Model file for the job. Use its own axes, mm. Give positions to 0.01 mm unless a question says otherwise; leave off trailing zeros. Write each loop counter-clockwise with the first axis right and the second up, starting at its lowest first coordinate (ties: lowest second). Pieces come first, ordered by that corner, then holes. Notation, with made-up numbers: (61, 62.5) - (119, 62.5) arc R28 cw to (119, 81.5) - close; hole circle Ø10 at (49.5, 23). An arc over 180 degrees is marked (long way). Use CSV: the item, a comma, the result in double quotes.
Autodesk Inventor part; units mm, degrees
ref_plane "Arbeitsebene7" through (120, 40, 0) normal (0, 1, 0) x (-1, 0, 0)
ref_plane "Arbeitsebene8" through (120, -40, 0) normal (0, 1, 0) x (-1, 0, 0)
ref_plane "Arbeitsebene10" through (20, -140, 0) normal (0, -1, 0) x (1, 0, 0)
sketch "Basis" plane through (0, 0, 0) normal (0, 0, 1) x (1, 0, 0)
  line L0 (0, 150) -> (0, -150)
  line L1 (-79.5351, 0) -> (153.2558, 0)
  line L2 (0, -282) -> (0, 222)
  line L3 (30, -50) -> (30, -210)
  line L4 (0, -200) -> (20, -200)
  line L5 (0, -40) -> (120, -40)
  line L6 (0, 40) -> (120, 40)
  line L7 (110, -30) -> (110, 30)
  point P0 (0, 0)
  point P1 (110, 0)
  dimension "d32" = 300
  dimension "d38" = 80
  dimension "d39" = 10
  dimension "d40" = 10
  dimension "d41" = 10
  dimension "d43" = 240
  dimension "d44" = 240
  dimension "d45" = 60
  dimension "d46" = 10
  dimension "d47" = 10
  dimension "d48" = 160
  dimension "d49" = 10
ref_plane "Arbeitsebene7" through (120, 40, 0) normal (0, 1, 0) x (-1, 0, 0)
sketch "Skizze12" plane through (120, 40, 0) normal (0, 1, 0) x (-1, 0, 0)
  line L0 (10, -10) -> (10, -80)
  line L1 (20, -70) -> (120, -70)
  line L2 (120, -100.8) -> (120, 16.8)
  point P0 (120, 0)
  point P1 (10, 0)
  point P2 (10, 0)
  point P3 (10, 0)
  dimension "d50" = 70
  dimension "d51" = 10
  dimension "d80" = 10
  dimension "d81" = 10
ref_plane "Arbeitsebene8" through (120, -40, 0) normal (0, 1, 0) x (-1, 0, 0)
sketch "Skizze13" plane through (120, -40, 0) normal (0, 1, 0) x (-1, 0, 0)
  line L0 (10, -10) -> (10, -80)
  line L1 (10, -10) -> (10, -80)
  line L2 (20, -70) -> (120, -70)
  line L3 (120, -100.8) -> (120, 16.8)
  point P0 (120, 0)
  dimension "d82" = 10
  dimension "d83" = 10
ref_plane "Arbeitsebene9" through (20, -200, 0) normal (0, -1, 0) x (1, 0, 0)
sketch "Skizze14" plane through (20, -200, 0) normal (0, -1, 0) x (1, 0, 0)
  line L0 (10, -10) -> (10, -50)
  point P0 (-20, 0)
  point P1 (10, 0)
  point P2 (10, 0)
  point P3 (10, 0)
  dimension "d52" = 40
  dimension "d53" = 10
ref_plane "Arbeitsebene10" through (20, -140, 0) normal (0, -1, 0) x (1, 0, 0)
sketch "Skizze15" plane through (20, -140, 0) normal (0, -1, 0) x (1, 0, 0)
  line L0 (10, -10) -> (10, -50)
  line L1 (10, -10) -> (10, -50)
  point P0 (-20, 0)
ref_plane "Arbeitsebene12" through (110, 40, -80) normal (1, 0, 0) x (0, 1, 0)
sketch "Skizze16" plane through (110, 40, -80) normal (1, 0, 0) x (0, 1, 0)
  line L0 (-90, 0) -> (10, 0)
  line L1 (10, 0) -> (10, -4)
  line L2 (10, -4) -> (-90, -4)
  line L3 (-90, -4) -> (-90, 0)
  line L4 (-70, 10) -> (-10, 10)
  line L5 (0, 70) -> (0, 0)
  line L6 (-80, 70) -> (-80, 0)
  point P0 (-40, 80)
  dimension "d66" = 4
  dimension "d67" = 10
  dimension "d68" = 10
  dimension "d77" = 10
  dimension "d78" = 10
  dimension "d79" = 10
ref_plane "Arbeitsebene17" through (110, -50, -84) normal (0, 0, 1) x (1, 0, 0)
sketch "Skizze18" plane through (110, -50, -84) normal (0, 0, 1) x (1, 0, 0)
  line L0 (-110, -232) -> (-110, 272)
  line L1 (-189.5351, 50) -> (43.2558, 50)
  line L2 (-19.5, 65.5) -> (-50.5, 65.5) construction
  line L3 (-50.5, 65.5) -> (-50.5, 34.5) construction
  line L4 (-19.5, 65.5) -> (-19.5, 34.5) construction
  line L5 (-19.5, 34.5) -> (-50.5, 34.5) construction
  point P0 (-110, 50)
  point P1 (-35, 50)
  dimension "d69" = 75
  dimension "d70" = 15.5
  dimension "d71" = 15.5
  dimension "d72" = 31
  dimension "d73" = 31
ref_plane "Arbeitsebene18" through (30, -140, -50) normal (1, 0, 0) x (0, 1, 0)
sketch "Skizze19" plane through (30, -140, -50) normal (1, 0, 0) x (0, 1, 0)
  line L0 (10, -4) -> (-70, -4)
  line L1 (-70, -4) -> (-70, 0)
  line L2 (-70, 0) -> (10, 0)
  line L3 (10, 0) -> (10, -4)
  line L4 (-50, 10) -> (-10, 10)
  point P0 (140, 50)
  point P1 (-60, 0)
  point P2 (0, 0)
  dimension "d74" = 4
  dimension "d75" = 10
  dimension "d76" = 10
  dimension "d84" = 10
  dimension "d85" = 10
  dimension "d86" = 10
ref_plane "Arbeitsebene19" through (30, -210, -54) normal (0, 0, 1) x (1, 0, 0)
ref_plane "Arbeitsebene20" through (20, 2.5, 100) normal (0, 0, -1) x (-1, 0, 0)
sketch "Skizze 1" plane through (-280, -73.3, 100) normal (0, 0, 1) x (1, 0, 0)
  line L0 (-20, 13.3) -> (-20, 11.3)
  line L1 (180, 13.3) -> (-20, 13.3)
  line L2 (180, -106.7) -> (-20, -106.7)
  line L3 (-20, -104.7) -> (-20, -106.7)
  line L4 (180, 53.3) -> (180, -146.7)
  line L5 (180, 73.3) -> (180, -166.7)
  line L6 (300, 73.3) -> (300, -166.7)
  line L7 (180, 73.3) -> (182, 73.3)
  line L8 (298, 73.3) -> (300, 73.3)
  line L9 (300, -166.7) -> (298, -166.7)
  line L10 (182, -166.7) -> (180, -166.7)
  line L11 (-20, -106.7) -> (-20, 13.3)
  line L12 (180, 13.3) -> (-20, 13.3)
  line L13 (180, 13.3) -> (180, 73.3)
  line L14 (180, 73.3) -> (300, 73.3)
  line L15 (300, -166.7) -> (300, 73.3)
  line L16 (300, -166.7) -> (180, -166.7)
  line L17 (180, -166.7) -> (180, -106.7)
  line L18 (180, -106.7) -> (-20, -106.7)
extrude "Extrusion3" add sketch "Skizze 1" along normal blind 10
sketch "Skizze23" plane through (20, -242.5, 0) normal (1, 0, 0) x (0, 0, -1)
  line L0 (0, 245) -> (0, 0)
  line L1 (-100, 245) -> (0, 245)
  line L2 (0, 0) -> (-100, 0)
  line L3 (-100, 0) -> (-100, 245)
  line L4 (-100, 245) -> (0, 245)
  line L5 (0, 245) -> (0, 0)
  point P0 (0, 242.5)
extrude "Extrusion4" cut sketch "Skizze23" against normal through all
sketch "Skizze20" plane through (30, -210, 100) normal (0, 0, 1) x (1, 0, 0)
  line L0 (0, 80) -> (0, 0)
  line L1 (-217.5819, 99.185) -> (-324.0785, 99.185) construction
  line L2 (-223.1225, 80.815) -> (-333.4519, 80.815) construction
  line L3 (-289.05, 125.855) -> (-289.05, 54.145) construction
  line L4 (-254.68, 148.5562) -> (-254.68, 51.145) construction
  line L5 (-44.2587, 170.5) -> (-93.3542, 170.5) construction
  line L6 (-85.5, 183.5563) -> (-85.5, 134.1968) construction
  line L7 (-97.1508, 139.5) -> (-51.7506, 139.5) construction
  line L8 (-54.5, 132.7748) -> (-54.5, 177.4853) construction
  line L9 (-327.4713, 90) -> (-3.4708, 90) construction
  line L10 (-70, 254.6178) -> (-70, -44.1957) construction
  line L11 (-130, 210) -> (-10, 210) construction
  line L12 (-330, 30) -> (-330, 150) construction
  circle A0 centre (-289.05, 99.185) radius 1.35
  circle A1 centre (-254.68, 99.185) radius 1.35
  circle A2 centre (-254.68, 80.815) radius 1.35
  circle A3 centre (-289.05, 80.815) radius 1.35
  circle A4 centre (-280, 90) radius 3
  circle A5 centre (-85.5, 170.5) radius 1.5
  circle A6 centre (-85.5, 139.5) radius 1.5
  circle A7 centre (-54.5, 139.5) radius 1.5
  circle A8 centre (-54.5, 170.5) radius 1.5
  circle A9 centre (-70, 155) radius 11
  point P0 (-30, 210)
  point P1 (-70, 210)
  point P2 (-330, 90)
  point P3 (-289.05, 90)
  dimension "d102" = 2.7
  dimension "d103" = 2.7
  dimension "d104" = 2.7
  dimension "d105" = 2.7
  dimension "d106" = 6
  dimension "d107" = 9.05
  dimension "d108" = 9.185
  dimension "d109" = 18.37
  dimension "d111" = 34.37
  dimension "d112" = 50
  dimension "d113" = 31
  dimension "d114" = 31
  dimension "d115" = 15.5
  dimension "d116" = 15.5
  dimension "d117" = 55
  dimension "d118" = 3
  dimension "d119" = 3
  dimension "d120" = 3
  dimension "d121" = 3
  dimension "d122" = 22
extrude "Extrusion5" cut sketch "Skizze20" along normal through all
ref_plane "Arbeitsebene21" through (-297.4713, -120, 100) normal (0, 1, 0) x (1, 0, 0)
mirror "Spiegeln1" about plane through (-297.4713, -120, 100) normal (0, 1, 0) of "Extrusion5"
fillet "Rundung1" radius 2 6 edges at (20, -240, 105) (20, 0, 105) (-100, 0, 105) (-300, -60, 105) (-300, -180, 105) (-100, -240, 105)
equation "\"d38\" = Bas_Haupt_Breite"
equation "\"d39\" = 0.5 * Alu_Prof"
equation "\"d40\" = d39"
equation "\"d41\" = d39"
equation "\"d43\" = Bas_Haupt_Länge + Alu_Prof"
equation "\"d44\" = d43"
equation "\"d45\" = Bas_Ver_Breite"
equation "\"d46\" = d39"
equation "\"d47\" = d39"
equation "\"d48\" = Bas_Ver_Länge"
equation "\"d49\" = d39"
equation "\"d50\" = Bas_Haupt_Höhe - 0.5 * Alu_Prof"
equation "\"d80\" = d51"
equation "\"d81\" = d51"
equation "\"d82\" = d81"
equation "\"d83\" = d81"
equation "\"d52\" = GM_Halt_Höhe - 0.5 * Alu_Prof"
equation "\"d66\" = Bas_Haupt_Plat_Höhe"
equation "\"d67\" = 0.5 * Alu_Prof"
equation "\"d68\" = d67"
equation "\"d77\" = d68"
equation "\"d78\" = d68"
equation "\"d79\" = d68"
equation "\"d70\" = 0.5 * SM_Schrauben_Pos_Abstand"
equation "\"d72\" = SM_Schrauben_Pos_Abstand"
equation "\"d73\" = SM_Schrauben_Pos_Abstand"
equation "\"d74\" = GM_Platte_Höhe"
equation "\"Zet_Kluppen_Höhe\" = 7"
equation "\"Zet_KluppenDicke\" = 1"
equation "\"Zet_Höhe\" = 5"
equation "\"Zet_Kluppen_Breite\" = 10"
equation "\"St_kurz_Breite\" = 10"
equation "\"Zet_Breite\" = 210"
equation "\"Gel_Mot_St_Breite\" = 10"
equation "\"Gel_Mot_St_2\" = 35"
equation "\"St_kurz_Höhe\" = 7.5"
equation "\"Gel_Mot_St_Höhe\" = 5"
equation "\"St_kurz_Länge\" = 140"
equation "\"St_lang_Länge\" = 180"
equation "\"Bas_Ver_Breite\" = 60"
equation "\"Bas_Ver_Länge\" = 160"
equation "\"Gel_Mot_St_1\" = 35"
equation "\"SM_Pos_Abstand\" = 150"
equation "\"GM_Halt_Höhe\" = 50"
equation "\"Bas_Haupt_Höhe\" = 80"
equation "\"Bas_Haupt_Breite\" = 80"
equation "\"Bas_Haupt_Länge\" = 220"
equation "\"Druck_teil_Höhe\" = 7.5"
equation "\"Druck_teil_Durchmesser\" = 50"
equation "\"Alu_Prof\" = 20"
equation "\"Bas_Haupt_Plat_Höhe\" = 4"
equation "\"SM_Scheibe_Durchmesser\" = 22"
equation "\"SM_Schrauben_Pos_Abstand\" = 31"
equation "\"GM_Platte_Höhe\" = 4"
equation "\"Rundung_Platte\" = 2"
equation "\"GM_Schrauben_Pos_Abstand_lang\" = 34.37"
equation "\"GM_Stift_Durchmesser\" = 6"
equation "\"GM_Schrauben_Pos_Abstand_kurz\" = 18.37"
equation "\"GM_Schrauben_Durchgangsloch\" = 2.7"
equation "\"GM_Schrauben_Pos_Stift_rlang\" = 9.05"
equation "\"GM_Schrauben_Pos_Stift_rkurz\" = 9.185"
properties part number "BT000_trajan20_21"
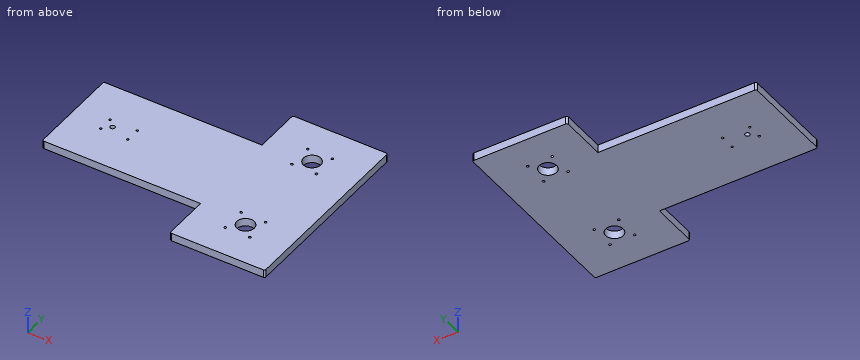
(1) Saw through at B-B, the plane z = 104. Count the separate pieces of the cut face and the enclosed holes in it, then the cut area to 3 significant figures.
Checked values:
separate pieces,"1"
enclosed holes,"15"
area,"51,900 mm^2"
(2) Flat gauge pins, fed straight in: P1, Ø6, axis at x = -103.5, z = 108.5, coming from the +Y side; P2, Ø5.5, axis at x = -250, y = -120, coming from the +Z side; P3, Ø2, axis at y = -209.5, z = 102, coming from the -X side; P4, Ø6, axis at x = -123.5, z = 103.5, coming from the -Y side. Where does each tip first touch, or does it go through?
Checked values:
P1,"stops at y = -60"
P2,"passes through"
P3,"stops at x = -100"
P4,"stops at y = -180"
(3) Saw through at A-A, the plane y = -185. List the corners of the cut face in (x, z).
Checked values:
outline,"(-100, 100) - (-51, 100) - (-51, 110) - (-100, 110) - close; (-29, 100) - (20, 100) - (20, 110) - (-29, 110) - close"
(4) Wall check: probe 1 along Y at (x, z) = (-224.68, 107.75) (3 decimals); probe 2 along X at (y, z) = (-39.5, 106); probe 3 along X at (y, z) = (-70.5, 105.25). Give the ranges that are in metal, low to high. Write a range as [from, to].
Checked values:
probe 1,"y = [-180, -130.535], [-127.835, -112.165], [-109.465, -60]"
probe 2,"x = [-100, -57], [-54, -26], [-23, 20]"
probe 3,"x = [-300, -57], [-54, -26], [-23, 20]"
(5) Saw through at C-C, the plane x = -138. List the corners of the cut face in (y, z), then the cut area to 3 significant figures.
Checked values:
outline,"(-180, 100) - (-60, 100) - (-60, 110) - (-180, 110) - close"
area,"1,200 mm^2"
